Check sheet for the drawn part. Datum: minimum x, y, z corner. Units: mm. A direction names the side the tool comes from. Round coordinates to 2 decimals unless told otherwise and drop trailing zeros. Loops run counter-clockwise (first coordinate to the right, second up) from the corner with the lowest first, then second, coordinate; pieces in that order, holes last.
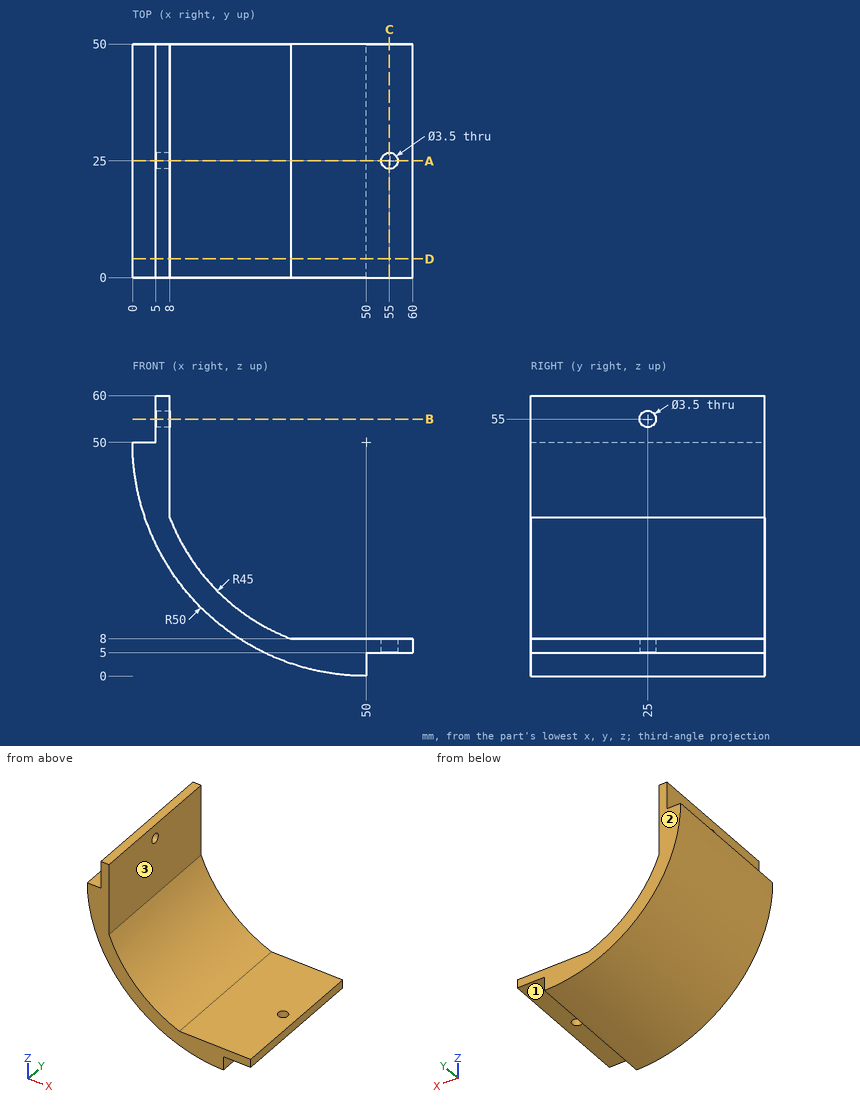
1) Sectioned sample at D-D, the plane y = 4. Record the cut outline in (x, z).
Report:
outline: (0, 50) arc R50 ccw to (50, 0) - (50, 5) - (60, 5) - (60, 8) - (33.84, 8) arc R45 cw to (8, 33.84) - (8, 60) - (5, 60) - (5, 50) - close
2) Sectioned sample at A-A, the plane y = 25. Record the cut outline in (x, z).
Report:
outline: (0, 50) arc R50 ccw to (50, 0) - (50, 5) - (53.25, 5) - (53.25, 8) - (33.84, 8) arc R45 cw to (8, 33.84) - (8, 53.25) - (5, 53.25) - (5, 50) - close; (5, 56.75) - (8, 56.75) - (8, 60) - (5, 60) - close; (56.75, 5) - (60, 5) - (60, 8) - (56.75, 8) - close
3) Sectioned sample at C-C, the plane x = 55. Record the cut outline in (y, z).
Report:
outline: (0, 5) - (23.25, 5) - (23.25, 8) - (0, 8) - close; (26.75, 5) - (50, 5) - (50, 8) - (26.75, 8) - close
4) Access from +Z, -Z, +X, -X, +Y, -Y to the whole of each face (thin tool, end or side, straight path). Record for the marked faces 1, 2 and 3.
Report:
face 1: -Z, +X, +Y, -Y
face 2: +Z, -Z, +X, -X, +Y
face 3: +Z, +X, +Y, -Y
5) Sectioned sample at B-B, the plane z = 55. Record the cut outline in (x, y).
Report:
outline: (5, 0) - (8, 0) - (8, 23.25) - (5, 23.25) - close; (5, 26.75) - (8, 26.75) - (8, 50) - (5, 50) - close
6) Scan lines: line 1 along Y through (x, z) = (55, 6.25); line 2 along Z through (x, y) = (53, 11.5); line 3 along X through (y, z) = (21.5, 38). Record each from-to range of solid material in increasing order.
Report:
line 1: y = 0 to 23.25, 26.75 to 50
line 2: z = 5 to 8
line 3: x = 1.46 to 8
7) Gauge pin test, flat ends, axial feed: pin 1 (2 mm diameter, centred on x = 55, y = 25, fed in from +Z); pin 2 (8 mm diameter, centred on x = 41.5, y = 14, fed in from +Z); pin 3 (3 mm diameter, centred on x = 55, y = 23.5, fed in from -Z); pin 4 (1.5 mm diameter, centred on x = 2.5, y = 25, fed in from +Z). Record the tip position at first contact, or that the pin passes through.
Report:
pin 1: passes through
pin 2: stops at z = 8
pin 3: stops at z = 5
pin 4: stops at z = 50
